The model under review builds one solid part; all positions refer to its coordinate system, in mm. A direction names the side the tool comes from. Coordinates: 2 decimals unless noted, no trailing zeros. Order: outer loops, then holes, each group sorted by start corner. A loop starts at its lowest first (then second) coordinate and runs counter-clockwise, first axis right, second up. Notation, with made-up numbers: M -19.75,-12 L 29.25,-12 A10 cw 29.25,5 Z; hole C 15.25,39.5 d6. An arc over 180 degrees is marked long. Write each question's results on one line, items separated by ' | '.
from build123d import *

# Parameters (mm, degrees)
M4X0_7_TAPPED_HOLE1_D     = 3.3
M4X0_7_TAPPED_HOLE1_DEPTH = 8.5
M4X0_7_TAPPED_HOLE1_TIP   = 0.991420021
CUT_EXTRUDE1_DEPTH        = 12.559411836
CUT_EXTRUDE1_DEPTH_BACK   = 12.559411836
SKETCH4_R                 = 1.25


with BuildPart() as part:
    # Sketch1 → Revolve1 (revolve)
    with BuildSketch(Plane.XY):
        with BuildLine():
            Line((0, 0), (-4.1, 0))
            Line((-4.1, 0), (-4.1, 1))
            Line((-4.1, 1), (-3.25, 1))
            Line((-3.25, 1), (-3.25, 4))
            add(Edge.make_bspline(
                [(-3.25, 4), (-3.25, 6.809673905), (-2.594523583, 8.691122547), (0, 10)],
                knots=[0, 0, 0, 0, 1, 1, 1, 1], degree=3))
            Line((0, 10), (0, 0))
        make_face()
    revolve(axis=Axis((0, 10, 0), (0, -1, 0)))

    # M4x0.7 Tapped Hole1
    with Locations(Plane(origin=(0, 0, 0), x_dir=(-1, 0, 0), z_dir=(0, -1, 0))):
        with Locations((0, 0)):
            Hole(M4X0_7_TAPPED_HOLE1_D / 2, depth=M4X0_7_TAPPED_HOLE1_DEPTH)
            with Locations((0, 0, -(M4X0_7_TAPPED_HOLE1_DEPTH + M4X0_7_TAPPED_HOLE1_TIP / 2))):  # 118° drill point
                Cone(0, M4X0_7_TAPPED_HOLE1_D / 2, M4X0_7_TAPPED_HOLE1_TIP, mode=Mode.SUBTRACT)

    # Sketch4 → Cut-Extrude1 (cut, two sides: drawn at the far end of the back side and taken through both)
    with BuildSketch(Plane.XY.offset(-CUT_EXTRUDE1_DEPTH_BACK)):
        with Locations((0, 6.5)):
            Circle(SKETCH4_R)
    extrude(amount=CUT_EXTRUDE1_DEPTH + CUT_EXTRUDE1_DEPTH_BACK, mode=Mode.SUBTRACT)


solid = part.part
1) The part is to be moulded in two halves that separate along Y. For faces 1 (the cylindrical face through (-0.27, 5.28, -2.15)), 2 (the flat face through (0, 0, 2)), 3 (the cylindrical face through (2.579, 2.521, 1.978)), say which applies: pulls with the +Y half, pulls with the -Y half, needs draft (parallel to the pull), parting line crosses it, or undercut.
Solutions:
face 1: undercut | face 2: pulls with the -Y half | face 3: needs draft
2) To check wall thickness, follow line 1 along Z through (x, y) = (0, 3.25); line 2 along Y through (x, z) = (0, -2.3); line 3 along X through (y, z) = (6.5, -1.9). State the ranges of each line that lie inside material, in increasing order.
Solutions:
line 1: -3.25 to -1.65, 1.65 to 3.25 | line 2: 0 to 5.25, 7.75 to 8.08 | line 3: -2.31 to -1.25, 1.25 to 2.31
3) Take a section at C-C on x = -3.5. State the section outline as (y, z) points, plus the area to 3 significant figures.
Solutions:
outline: M 0,-2.14 L 1,-2.14 L 1,2.14 L 0,2.14 Z | area: 4.27 mm2
4) Take a section at A-A on y = 2. State the section outline as (x, z) points.
Solutions:
outline: C 0,0 d6.5; hole C 0,0 d3.3
5) For faces 4 (the cylindrical face through (-1.65, 4.31, -0.07)), 5 (the flat face through (3, 1, -2)), 6 (the cylindrical face through (0.534, 0.507, -4.065)), list the 3-axis set-ups (+Z, -Z, +X, -X, +Y, -Y) from which the entire face can be reached by the end or side of a thin tool; tool diameter is ignored.
Solutions:
face 4: -Y | face 5: +Y | face 6: +Y, -Y
6) Take a section at B-B on x = -0.25. Count the separate pieces of the cut face and the enclosed holes in it, plus the area to 3 significant figures.
Solutions:
separate pieces: 3 | enclosed holes: 0 | area: 21.4 mm2
7) Take a section at D-D on x = 3.75. State the section outline as (y, z) points, plus the area to 3 significant figures.
Solutions:
outline: M 0,-1.66 L 1,-1.66 L 1,1.66 L 0,1.66 Z | area: 3.32 mm2
8) For pin 1 (1.5 mm diameter, centred on x = 3, y = 6.5, fed in from +Z); pin 2 (3 mm diameter, centred on x = 0, y = 6.5, fed in from +Z); pin 3 (1.5 mm diameter, centred on x = 1.5, y = 5, fed in from -Z); pin 4 (2 mm diameter, centred on x = 0, y = 6.5, fed in from -Z), all flat-tipped, find the tip position at first contact; note any pin that passes through.
Solutions:
pin 1: z = 2.01 | pin 2: z = 3.22 | pin 3: z = -3.14 | pin 4: through
